from build123d import *

# Parameters (mm, degrees)
SKETCH1_W           = 50
SKETCH1_H           = 16.582990108
SKETCH1_R           = 5
BOSS_EXTRUDE1_DEPTH = 10
SKETCH2_R           = 5
BOSS_EXTRUDE2_DEPTH = 32.5158
SKETCH3_R           = 1.75
CUT_EXTRUDE1_DEPTH  = 10


with BuildPart() as part:
    # Sketch1 → Boss-Extrude1 (new body)
    with BuildSketch(Plane(origin=(0, 0, 0), x_dir=(1, 0, 0), z_dir=(0, 1, 0))):
        with Locations((9.061664817, 20.692573909)):
            Rectangle(SKETCH1_W, SKETCH1_H)
        with Locations((1.261664817, 19.401078855)):
            Circle(SKETCH1_R, mode=Mode.SUBTRACT)
        with Locations((17.061664817, 19.401078855)):
            Circle(SKETCH1_R, mode=Mode.SUBTRACT)
    extrude(amount=BOSS_EXTRUDE1_DEPTH)

    # Sketch2 → Boss-Extrude2 (add)
    with BuildSketch(Plane.XZ):
        with Locations((28.061664817, -21.004215915)):
            Circle(SKETCH2_R)
        with Locations((-9.938335183, -21.004215915)):
            Circle(SKETCH2_R)
    extrude(amount=BOSS_EXTRUDE2_DEPTH)

    # Sketch3 → Cut-Extrude1 (cut)
    with BuildSketch(Plane.XZ.offset(32.5158)):
        with Locations((28.061664817, -21.004215915)):
            Circle(SKETCH3_R)
        with Locations((-9.938335183, -21.004215915)):
            Circle(SKETCH3_R)
    extrude(amount=-CUT_EXTRUDE1_DEPTH, mode=Mode.SUBTRACT)


solid = part.part
Input: part model. Units: mm. Frame: model coordinates. A direction names the side the tool comes from. Coordinates: 2 decimals unless noted, no trailing zeros. Order: outer loops, then holes, each group sorted by start corner. A loop starts at its lowest first (then second) coordinate and runs counter-clockwise, first axis right, second up. Notation, with made-up numbers: M 62,44.5 L 91,44.5 A7 cw 91,51.5 Z; hole C 68,70.5 d1. An arc over 180 degrees is marked long. Answer in a Markdown table with one row per item.
(1) Section query B-B, the plane z = -23.5. Output: boundary loops of the cut face in (x, y).
Numbers:
| item | result |
|---|---|
| outline | M -15.94,0 L -14.27,0 L -14.27,-32.52 L -5.61,-32.52 L -5.61,0 L -1.6,0 L -1.6,10 L -15.94,10 Z; M 4.13,0 L 14.2,0 L 14.2,10 L 4.13,10 Z; M 19.93,0 L 23.73,0 L 23.73,-32.52 L 32.39,-32.52 L 32.39,0 L 34.06,0 L 34.06,10 L 19.93,10 Z |
(2) Access query for faces 5 (the flat face through (9, 10, -21)), 6 (the flat face through (28, -22.516, -21)). Directions: +Z, -Z, +X, -X, +Y, -Y. A direction counts if a zero-diameter tool reaches every point of the face in a straight line with its end or side. Return the directions, or none.
Numbers:
| item | result |
|---|---|
| face 5 | +Z, -Z, +X, -X, +Y |
| face 6 | -Y |
(3) Section query C-C, the plane y = 1. Output: boundary loops of the cut face in (x, z).
Numbers:
| item | result |
|---|---|
| outline | M -15.94,-28.98 L 34.06,-28.98 L 34.06,-12.4 L -15.94,-12.4 Z; hole C 1.26,-19.4 d10; hole C 17.06,-19.4 d10 |
(4) Section query A-A, the plane x = 2.5. Output: boundary loops of the cut face in (y, z).
Numbers:
| item | result |
|---|---|
| outline | M 0,-28.98 L 10,-28.98 L 10,-24.25 L 0,-24.25 Z; M 0,-14.56 L 10,-14.56 L 10,-12.4 L 0,-12.4 Z |
(5) Section query D-D, the plane x = 11. Output: boundary loops of the cut face in (y, z).
Numbers:
| item | result |
|---|---|
| outline | M 0,-28.98 L 10,-28.98 L 10,-12.4 L 0,-12.4 Z |
(6) Contact query for flat-ended pins moving along their axis: pin 1 Ø4 at (y, z) = (-16, -21.5) entering from +X; pin 2 Ø5 at (y, z) = (-21, -22.5) entering from -X; pin 3 Ø1 at (x, z) = (29, -21) entering from -Y; pin 4 Ø3 at (x, z) = (-9.5, -21) entering from -Y. Output: stop coordinate, or through.
Numbers:
| item | result |
|---|---|
| pin 1 | stops at x = 33.06 |
| pin 2 | stops at x = -14.94 |
| pin 3 | stops at y = -22.52 |
| pin 4 | stops at y = -32.52 |
(7) Material intervals for line 1 (X direction, y = 6, z = -17); line 2 (X direction, y = 2.5, z = -21.5); line 3 (X direction, y = -29, z = -19.75), sorted ascending. Write a range as [from, to].
Numbers:
| item | result |
|---|---|
| line 1 | x = [-15.94, -3.12], [5.65, 12.68], [21.45, 34.06] |
| line 2 | x = [-15.94, -3.28], [5.8, 12.52], [21.6, 34.06] |
| line 3 | x = [-14.78, -11.16], [-8.72, -5.1], [23.22, 26.84], [29.28, 32.9] |
(8) Draft query along Z for faces 1 (the cylindrical face through (-10.17, -27.59, -19.27)), 2 (the flat face through (9, 5, -28.984)), 3 (the flat face through (-15.938, 5, -21)), 4 (the cylindrical face through (24.094, -16.03, -24.047)). Return one class per face: pulls with the +Z half, pulls with the -Z half, needs draft (parallel to the pull), parting line crosses it, or undercut.
Numbers:
| item | result |
|---|---|
| face 1 | undercut |
| face 2 | pulls with the -Z half |
| face 3 | needs draft |
| face 4 | parting line crosses it |
